Here's how the part is built. I have some questions about the finished solid (model axes, mm). Face numbers are marked on the shaded views. Coordinates: 2 decimals unless noted, no trailing zeros. Write each loop counter-clockwise with the first axis right and the second up, starting at its lowest first coordinate (ties: lowest second). Pieces come first, ordered by that corner, then holes. Notation, with made-up numbers: (51.5, 24) -> (77.5, 24) arc R22 ccw to (77.5, 54) -> close; hole circle Ø11 at (43, 43). An arc over 180 degrees is marked (long way). Use a Markdown table: item, result. Add a question column.
Item 1: If I drill on line 1 along Y through (x, z) = (-19, -112); line 2 along Z through (x, y) = (-130.5, 28.5); line 3 along Z through (x, y) = (-187.5, 17.5), over which ranges is the centre line in solid material (lowest first)? Write a range as from..to.
Item 2: Imagine slicing it at A-A, the plane y = 19.05. Write out the boundary of the cut face in (x, z) (3 decimals), and give its area (3 significant figures).
Item 3: If we mould it in two halves opening along Z, with no side actions, what happens to the marked faces 1, 2, 3 and 4? For each: pulls with the +Z half, pulls with the -Z half, needs draft (parallel to the pull), parting line crosses it, or undercut.
Item 4: Will these pins go through, and if not, where does the flat tip stop? pin 1 Ø6 at (x, y) = (-342, 13.5) entering from +Z (3 decimals); pin 2 Ø7.5 at (y, z) = (17.5, 12) entering from -X; pin 3 Ø5 at (x, y) = (-308.5, 23.5) entering from +Z (3 decimals); pin 4 Ø15 at (x, y) = (-19.05, 19.05) entering from -Z.
Item 5: Imagine slicing it at B-B, the plane x = -19.05. Write out the boundary of the cut face in (y, z) (3 decimals), and give its area (3 significant figures).
Item 6: Imagine slicing it at C-C, the plane x = -373. Write out the boundary of the cut face in (y, z) (3 decimals), and give its area (3 significant figures).
Item 7: Imagine slicing it at D-D, the plane z = -82.5. Write out the boundary of the cut face in (x, y).
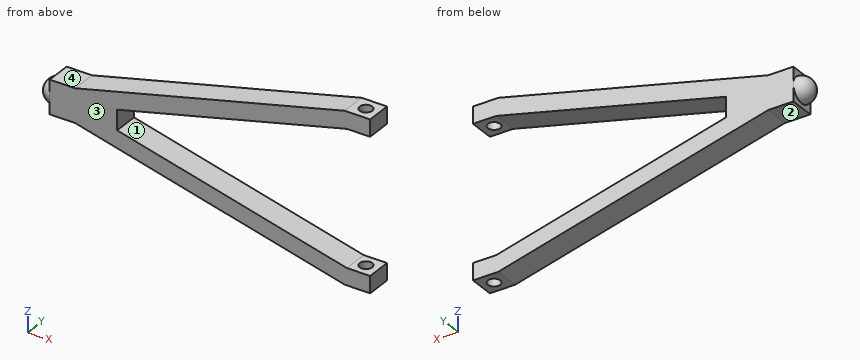
```python
from build123d import *

# Parameters (mm, degrees)
BOSS_EXTRUDE1_DEPTH     = 38.1
CUT_EXTRUDE1_DEPTH      = 564.578151191
CUT_EXTRUDE1_DEPTH_BACK = 564.578151191
SKETCH3_R               = 9.525


# Read off the part's stored shape, not the designer's step: Revolve1
with BuildPart() as part:
    # Sketch1 → Boss-Extrude1 (new body)
    with BuildSketch(Plane(origin=(0, 0, 0), x_dir=(1, 0, 0), z_dir=(0, 1, 0))):
        Polygon((-38.1, 127), (-444.5, 25.4), (-482.6, 25.4), (-482.6, -25.4), (-444.5, -25.4), (-38.1, -127), (0, -127), (0, -101.6), (-34.973117109, -101.6), (-381, -15.093279277), (-381, 15.093279277), (-34.973117109, 101.6), (0, 101.6), (0, 127), align=None)
    extrude(amount=BOSS_EXTRUDE1_DEPTH)

    # Revolve1 outline → Revolve1 (revolve)
    with BuildSketch(Plane(origin=(0, 19.05, 0), x_dir=(0, 1, 0), z_dir=(0, 0, -1))):
        with BuildLine():
            Line((0, -482.599999981), (0, -501.65))
            ThreePointArc((0, -501.65), (13.470384188, -496.070384175), (19.05, -482.599999981))
            Line((19.05, -482.599999981), (0, -482.599999981))
        make_face()
    revolve(axis=Axis((0, 19.05, 0), (1, 0, 0)))

    # Sketch3 → Cut-Extrude1 (cut, two sides: drawn at the far end of the back side and taken through both)
    with BuildSketch(Plane.XY.offset(127).offset(-CUT_EXTRUDE1_DEPTH_BACK)):
        with Locations((-19.05, 19.05)):
            Circle(SKETCH3_R)
    extrude(amount=CUT_EXTRUDE1_DEPTH + CUT_EXTRUDE1_DEPTH_BACK, mode=Mode.SUBTRACT)


solid = part.part
```
Ans:
| question | item | result |
|---|---|---|
| 1 | line 1 | y = 0..9.53, 28.57..38.1 |
| 1 | line 2 | z = -103.9..-77.72, 77.72..103.9 |
| 1 | line 3 | z = -89.65..-63.47, 63.47..89.65 |
| 2 | outline | (-482.6, -25.4) -> (-444.5, -25.4) -> (-38.1, -127) -> (-28.575, -127) -> (-28.575, -101.6) -> (-34.973, -101.6) -> (-381, -15.093) -> (-381, 15.093) -> (-34.973, 101.6) -> (-28.575, 101.6) -> (-28.575, 127) -> (-38.1, 127) -> (-444.5, 25.4) -> (-482.6, 25.4) -> (-482.6, 19.05) arc R19.05 ccw to (-482.6, -19.05) -> close; (-9.525, -127) -> (0, -127) -> (0, -101.6) -> (-9.525, -101.6) -> close; (-9.525, 101.6) -> (0, 101.6) -> (0, 127) -> (-9.525, 127) -> close |
| 2 | area | 25,700 mm^2 |
| 3 | face 1 | undercut |
| 3 | face 2 | pulls with the -Z half |
| 3 | face 3 | needs draft |
| 3 | face 4 | pulls with the +Z half |
| 4 | pin 1 | stops at z = 51.775 |
| 4 | pin 2 | stops at x = -499.72 |
| 4 | pin 3 | stops at z = 60.025 |
| 4 | pin 4 | passes through |
| 5 | outline | (0, -127) -> (9.525, -127) -> (9.525, -101.6) -> (0, -101.6) -> close; (0, 101.6) -> (9.525, 101.6) -> (9.525, 127) -> (0, 127) -> close; (28.575, -127) -> (38.1, -127) -> (38.1, -101.6) -> (28.575, -101.6) -> close; (28.575, 101.6) -> (38.1, 101.6) -> (38.1, 127) -> (28.575, 127) -> close |
| 5 | area | 968 mm^2 |
| 6 | outline | (0, -43.275) -> (38.1, -43.275) -> (38.1, -17.093) -> (0, -17.093) -> close; (0, 17.093) -> (38.1, 17.093) -> (38.1, 43.275) -> (0, 43.275) -> close |
| 6 | area | 2,000 mm^2 |
| 7 | outline | (-216.1, 0) -> (-111.37, 0) -> (-111.37, 38.1) -> (-216.1, 38.1) -> close |
